```python
from build123d import *

# Parameters (mm, degrees)
BOSS_EXTRUDE1_DEPTH = 120
SKETCH2_R           = 2.9
CUT_EXTRUDE1_DEPTH  = 4
SKETCH3_R           = 1.7
CUT_EXTRUDE2_DEPTH  = 121.403488322


with BuildPart() as part:
    # Sketch1 → Boss-Extrude1 (new body)
    with BuildSketch(Plane.XY):
        Polygon((9, 6.4), (9, 4.9), (8.2, 4.45), (9, 4), (9, 0), (0, 0), (0, 4), (0.8, 4.45), (0, 4.9), (0, 6.4), align=None)
    extrude(amount=BOSS_EXTRUDE1_DEPTH)

    # Sketch2 → Cut-Extrude1 (cut)
    with BuildSketch(Plane(origin=(0, 6.4, 0), x_dir=(1, 0, 0), z_dir=(0, 1, 0))):
        with Locations(Location((4.5, -110, 0), (0, 0, 270))):
            Circle(SKETCH2_R)
        with Locations(Location((4.5, -90, 0), (0, 0, 270))):
            Circle(SKETCH2_R)
        with Locations(Location((4.5, -70, 0), (0, 0, 270))):
            Circle(SKETCH2_R)
        with Locations(Location((4.5, -50, 0), (0, 0, 270))):
            Circle(SKETCH2_R)
        with Locations(Location((4.5, -30, 0), (0, 0, 270))):
            Circle(SKETCH2_R)
        with Locations(Location((4.5, -10, 0), (0, 0, 270))):
            Circle(SKETCH2_R)
        with Locations((4.5, 10)):
            Circle(SKETCH2_R)
    extrude(amount=-CUT_EXTRUDE1_DEPTH, mode=Mode.SUBTRACT)

    # Sketch3 → Cut-Extrude2 (cut, through all)
    with BuildSketch(Plane(origin=(0, 2.4, 0), x_dir=(1, 0, 0), z_dir=(0, 1, 0))):
        with Locations(Location((4.5, -110, 0), (0, 0, 270))):
            Circle(SKETCH3_R)
        with Locations(Location((4.5, -90, 0), (0, 0, 270))):
            Circle(SKETCH3_R)
        with Locations(Location((4.5, -70, 0), (0, 0, 270))):
            Circle(SKETCH3_R)
        with Locations(Location((4.5, -50, 0), (0, 0, 270))):
            Circle(SKETCH3_R)
        with Locations(Location((4.5, -30, 0), (0, 0, 270))):
            Circle(SKETCH3_R)
        with Locations(Location((4.5, -10, 0), (0, 0, 270))):
            Circle(SKETCH3_R)
        with Locations((4.5, 10)):
            Circle(SKETCH3_R)
    extrude(amount=-CUT_EXTRUDE2_DEPTH, mode=Mode.SUBTRACT)


solid = part.part
```
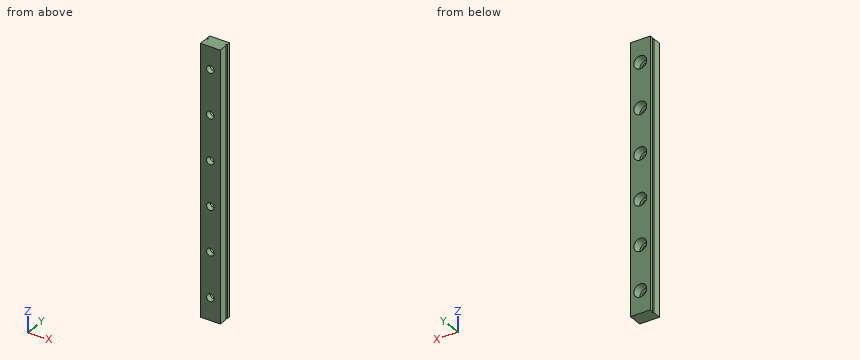
For this review, take the finished solid that the model builds, in its own axes (mm). Give positions to 0.01 mm unless a question says otherwise; leave off trailing zeros. Write each loop counter-clockwise with the first axis right and the second up, starting at its lowest first coordinate (ties: lowest second). Pieces come first, ordered by that corner, then holes.
Item 1: Take a section at B-B (x = 4.5). Give the number of separate pieces and of enclosed holes in the cut face, and give its area (3 significant figures).
Item 2: Take a section at A-A (z = 30). Give the boundary of the cut face in (x, y), and give its area (3 significant figures).
Item 3: Wall thickness on probe 1 along X at (y, z) = (3.65, 30); probe 2 along Y at (x, z) = (3.25, 88.5); probe 3 along Y at (x, z) = (0.5, 18): over which ranges is each line inside the solid? List them lowest first.
Item 4: Insertion check: P1, Ø1.5, axis at x = 3, z = 98.5, coming from the -Y side; P2, Ø4.5, axis at x = 5, z = 110, coming from the +Y side; P3, Ø2, axis at x = 4.5, z = 110, coming from the +Y side. Each pin has a flat end and moves straight along its axis. Give the tip position at first contact, or say it passes through.
Established:
1. separate pieces: 7
1. enclosed holes: 0
1. area: 580 mm2
2. outline: (0, 0) - (2.8, 0) - (2.8, 2.4) - (1.6, 2.4) - (1.6, 6.4) - (0, 6.4) - (0, 4.9) - (0.8, 4.45) - (0, 4) - close; (6.2, 0) - (9, 0) - (9, 4) - (8.2, 4.45) - (9, 4.9) - (9, 6.4) - (7.4, 6.4) - (7.4, 2.4) - (6.2, 2.4) - close
2. area: 25.5 mm2
3. probe 1: x = 0 to 1.6, 7.4 to 9
3. probe 2: y = 0 to 2.4
3. probe 3: y = 0 to 4.28, 4.62 to 6.4
4. P1: stops at y = 0
4. P2: stops at y = 2.4
4. P3: passes through
